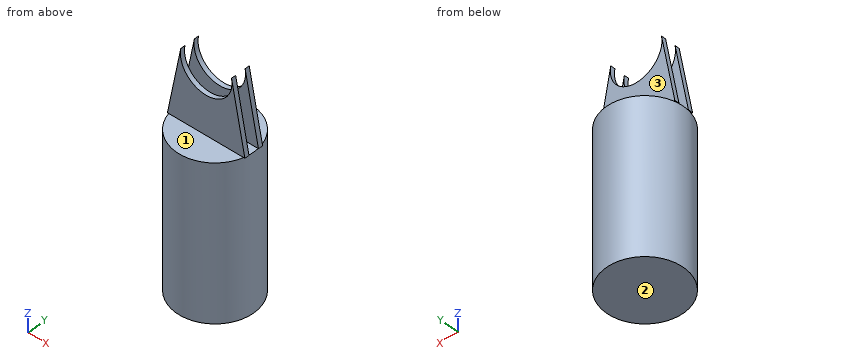
from build123d import *

# Parameters (mm, degrees)
POLE_SKETCH_R                   = 30
POLE_EXTRUDE_DEPTH              = 120
UPPER_START                     = 4
UPPER_PALM_HOLDER_EXTRUDE_DEPTH = 3.5
LOWER_START                     = -7.5
LOWER_PALM_HOLDER_EXTRUDE_DEPTH = 3.5


with BuildPart() as part:
    # Pole Sketch → Pole Extrude (new body)
    with BuildSketch(Plane.XY):
        Circle(POLE_SKETCH_R)
    extrude(amount=-POLE_EXTRUDE_DEPTH)

    # Palm Holder Sketch → Upper Palm Holder Extrude (add)
    with BuildSketch(Plane(origin=(0, 0, 0), x_dir=(1, 0, 0), z_dir=(0, 1, 0)).offset(UPPER_START)):
        with BuildLine():
            Line((19.63889875, -53.78333925), (30, 0))
            Line((30, 0), (-30, 0))
            Line((-30, 0), (-19.63889875, -53.78333925))
            ThreePointArc((-19.63889875, -53.78333925), (0, -30), (19.63889875, -53.78333925))
        make_face()
    extrude(amount=UPPER_PALM_HOLDER_EXTRUDE_DEPTH)

    # Palm Holder Sketch<2> → Lower Palm Holder Extrude (add)
    with BuildSketch(Plane(origin=(0, 0, 0), x_dir=(1, 0, 0), z_dir=(0, 1, 0)).offset(LOWER_START)):
        with BuildLine():
            Line((19.63889875, -53.78333925), (30, 0))
            Line((30, 0), (-30, 0))
            Line((-30, 0), (-19.63889875, -53.78333925))
            ThreePointArc((-19.63889875, -53.78333925), (0, -30), (19.63889875, -53.78333925))
        make_face()
    extrude(amount=LOWER_PALM_HOLDER_EXTRUDE_DEPTH)


solid = part.part
Work out the finished part from the listing and answer in its coordinate system (mm). Face numbers are marked on the shaded views. A direction names the side the tool comes from. Coordinates: 2 decimals unless noted, no trailing zeros. Write each loop counter-clockwise with the first axis right and the second up, starting at its lowest first coordinate (ties: lowest second). Pieces come first, ordered by that corner, then holes. Notation, with made-up numbers: M 76,27 L 121,27 A33 cw 121,61 Z; hole C 89,-11.75 d11. An arc over 180 degrees is marked long. Use one line per item in the form item = value. Start each with the question number.
1. Each of these flat-tipped pins is pushed along its axis until it touches: P1, Ø3, axis at y = -6, z = -4, coming from the -X side; P2, Ø4, axis at y = 15.5, z = -7.5, coming from the +X side; P3, Ø6.5, axis at x = -10.5, y = 0, coming from the +Z side; P4, Ø1, axis at x = 29.5, y = -6.5, coming from the -Z side. Where does it stop, or does it pass through?
2. The part is cut by section A-A (x = 0). Give the vertices of the cut face in (y, z).
3. The part is cut by section D-D (y = 0). Give the vertices of the cut face in (x, z).
4. The part is cut by section B-B (z = 15.5). Give the vertices of the cut face in (x, y), plus the area to 3 significant figures.
5. A tool of negligible diameter and unlimited length cuts with its end or side. For the marked faces 1, 2 and 3, from which of +Z, -Z, +X, -X, +Y, -Y can it reach the whole face along a straight path? Write none if from no direction.
6. Straight lines are drawn through the part: probe 1 along Y at (x, z) = (9.5, 29); probe 2 along Z at (x, y) = (0, -6); probe 3 along Z at (x, y) = (4, 15.5). For each, find the intervals that lie inside material, in ascending order. Write a range as from..to.
7. The part is cut by section C-C (z = 50). Give the vertices of the cut face in (x, y).
Evaluation:
q1.P1 = -29.66
q1.P2 = 26.79
q1.P3 = 0
q1.P4 = -120
q2.outline = M -30,-120 L 30,-120 L 30,0 L 7.5,0 L 7.5,30 L 4,30 L 4,0 L -4,0 L -4,30 L -7.5,30 L -7.5,0 L -30,0 Z
q3.outline = M -30,-120 L 30,-120 L 30,0 L -30,0 Z
q4.outline = M -27.01,-7.5 L 27.01,-7.5 L 27.01,-4 L -27.01,-4 Z; M -27.01,4 L 27.01,4 L 27.01,7.5 L -27.01,7.5 Z
q4.area = 378 mm^2
q5.face_1 = +Z, +X, -X, -Y
q5.face_2 = -Z, +X, -X, +Y, -Y
q5.face_3 = +Z, +X, -X, +Y
q6.probe_1 = -7.5..-4, 4..7.5
q6.probe_2 = -120..30
q6.probe_3 = -120..0
q7.outline = M -20.37,-7.5 L -20,-7.5 L -20,-4 L -20.37,-4 Z; M -20.37,4 L -20,4 L -20,7.5 L -20.37,7.5 Z; M 20,-7.5 L 20.37,-7.5 L 20.37,-4 L 20,-4 Z; M 20,4 L 20.37,4 L 20.37,7.5 L 20,7.5 Z
